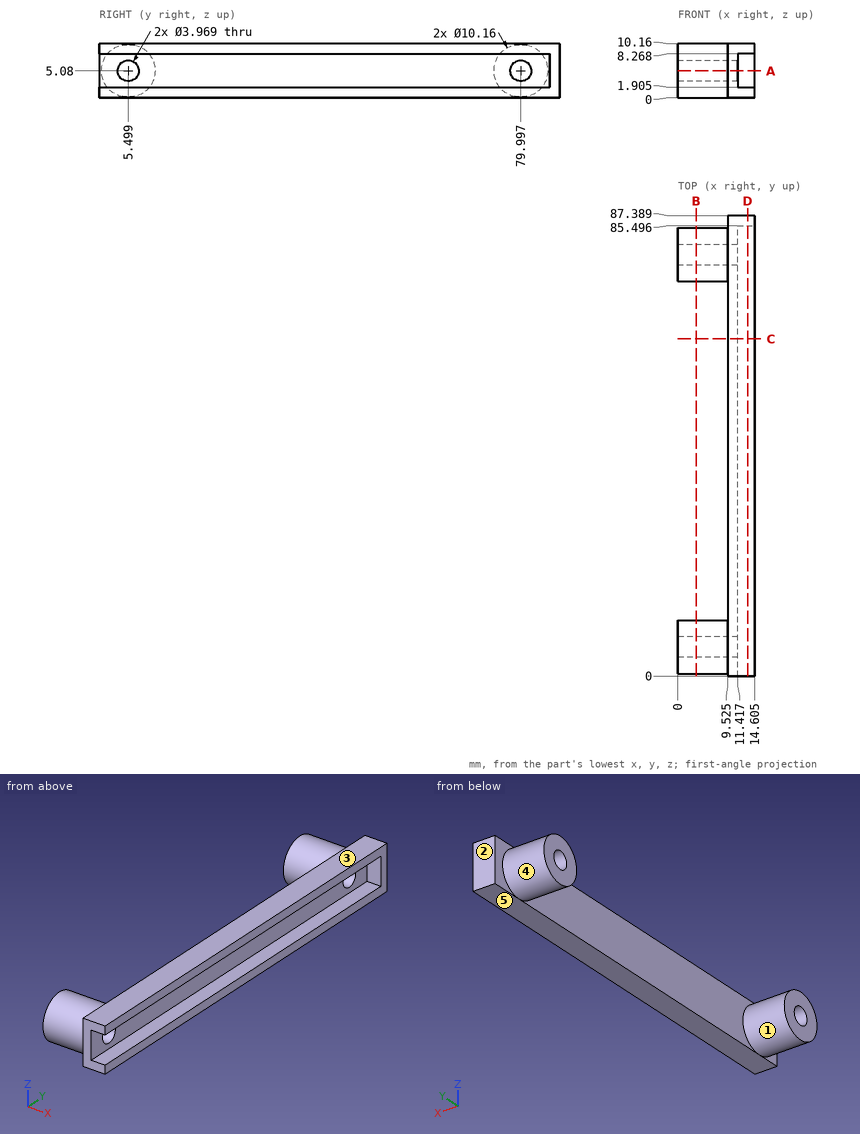
Check sheet for the drawn part. Datum: minimum x, y, z corner. Units: mm. A direction names the side the tool comes from. Give positions to 0.01 mm unless a question says otherwise; leave off trailing zeros. Write each loop counter-clockwise with the first axis right and the second up, starting at its lowest first coordinate (ties: lowest second). Pieces come first, ordered by that corner, then holes. Notation, with made-up numbers: M 6.5,18.5 L 20.5,18.5 A23 ccw 20.5,50.5 Z; hole C -10,16.25 d4. An arc over 180 degrees is marked long. Write item = value, one per line.
(1) Sectioned sample at C-C (y = 64). Record the cut outline in (x, z) (1 decimal).
Found:
outline = M 9.5,0 L 14.6,0 L 14.6,1.9 L 11.4,1.9 L 11.4,8.3 L 14.6,8.3 L 14.6,10.2 L 9.5,10.2 Z
(2) Sectioned sample at D-D (x = 13.25). Record the cut outline in (y, z) (1 decimal), then the cut area to 3 significant figures.
Found:
outline = M 0,0 L 87.4,0 L 87.4,10.2 L 0,10.2 L 0,8.3 L 85.5,8.3 L 85.5,1.9 L 0,1.9 Z
area = 344 mm2
(3) Material ranges on line 1 (Y direction, x = 7.25, z = 5.08) (1 decimal); line 2 (Z direction, x = 12.75, y = 44.5) (1 decimal); line 3 (Y direction, x = 7.5, z = 5.75) (1 decimal), recorded low to high.
Found:
line_1 = 0.4 to 3.5, 7.5 to 10.6, 74.9 to 78, 82 to 85.1
line_2 = 0 to 1.9, 8.3 to 10.2
line_3 = 0.5 to 3.6, 7.4 to 10.5, 75 to 78.1, 81.9 to 85
(4) Sectioned sample at B-B (x = 3.5). Record the cut outline in (y, z) (1 decimal).
Found:
outline = C 5.5,5.1 d10.2; C 80,5.1 d10.2; hole C 5.5,5.1 d4; hole C 80,5.1 d4
(5) Sectioned sample at A-A (z = 5.08). Record the cut outline in (x, y) (1 decimal).
Found:
outline = M 0,0.4 L 9.5,0.4 L 9.5,0 L 11.4,0 L 11.4,3.5 L 0,3.5 Z; M 0,7.5 L 11.4,7.5 L 11.4,78 L 0,78 L 0,74.9 L 9.5,74.9 L 9.5,10.6 L 0,10.6 Z; M 0,82 L 11.4,82 L 11.4,85.5 L 14.6,85.5 L 14.6,87.4 L 9.5,87.4 L 9.5,85.1 L 0,85.1 Z
(6) Draft check along Y on the marked faces 1, 2 and 3. Enter one of: released by +Y, released by -Y, zero draft, split by the parting line, or undercut.
Found:
face_1 = undercut
face_2 = released by +Y
face_3 = zero draft
(7) Go/stop test with flat-tipped pins: pin 1 Ø2 at (y, z) = (17.5, 1.5) entering from -X (3 decimals); pin 2 Ø2.5 at (x, z) = (13.5, 5) entering from -Y; pin 3 Ø2 at (y, z) = (62, 4.5) entering from +X. Record where each tip stops, or that it passes through.
Found:
pin_1 = 9.525
pin_2 = 85.5
pin_3 = 11.42
(8) Access from +Z, -Z, +X, -X, +Y, -Y to the whole of each face (thin tool, end or side, straight path). Record for the marked faces 4 and 5.
Found:
face_4 = -X
face_5 = -Z, +X, -X, +Y, -Y
